Drawing for the job (mm, zero at the part's lowest x, y, z). A direction names the side the tool comes from. Coordinates: 2 decimals unless noted, no trailing zeros. Order: outer loops, then holes, each group sorted by start corner. A loop starts at its lowest first (then second) coordinate and runs counter-clockwise, first axis right, second up. Notation, with made-up numbers: M 25,30 L 64,30 A16 ccw 64,57 Z; hole C 78.25,20 d6. An arc over 180 degrees is marked long. Write item = value, one per line. Start each with the question number.
Q1. Drill centre lines: probe 1 along Z at (x, y) = (13.5, 27); probe 2 along Z at (x, y) = (34, 10.25); probe 3 along X at (y, z) = (12.5, 18). Where is each one in solid material? Low to high.
Q2. Band-saw the part on C-C on z = 28. Write the cut outline in (x, y), plus the area to 3 significant figures.
Q3. Band-saw the part on D-D on x = 4. Write the cut outline in (y, z).
Q4. Pin check, flat tips, straight feed: P1, Ø6, axis at y = 14, z = 14.5, coming from the -X side; P2, Ø7.5, axis at x = 22, z = 27.5, coming from the +Y side; P3, Ø10, axis at x = 18.5, y = 24.5, coming from the +Z side. Stop position of each tip, or through.
Q5. Band-saw the part on B-B on y = 18. Write the cut outline in (x, z).
Q6. 3-axis set-ups, long thin cutter, end or side, ignore diameter. For the marked faces 1, 2 and 3: which of +Z, -Z, +X, -X, +Y, -Y reach the whole face in a straight line?
Q7. Band-saw the part on A-A on x = 35.5. Write the cut outline in (y, z).
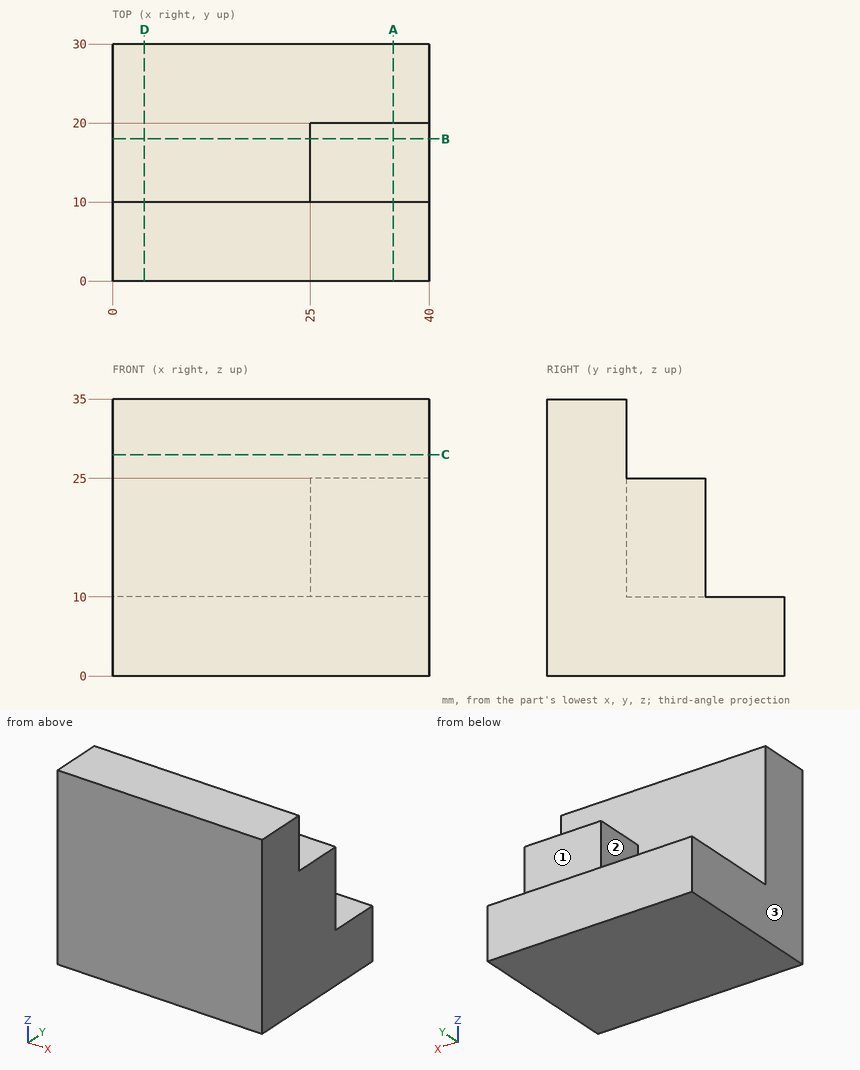
Recorded:
q1.probe_1 = 0 to 10
q1.probe_2 = 0 to 25
q1.probe_3 = 25 to 40
q2.outline = M 0,0 L 40,0 L 40,10 L 0,10 Z
q2.area = 400 mm2
q3.outline = M 0,0 L 30,0 L 30,10 L 10,10 L 10,35 L 0,35 Z
q4.P1 = 25
q4.P2 = 10
q4.P3 = 10
q5.outline = M 0,0 L 40,0 L 40,25 L 25,25 L 25,10 L 0,10 Z
q6.face_1 = +Z, +X, -X, +Y
q6.face_2 = +Z, -X, +Y
q6.face_3 = +Z, -Z, -X, +Y, -Y
q7.outline = M 0,0 L 30,0 L 30,10 L 20,10 L 20,25 L 10,25 L 10,35 L 0,35 Z
